Job drawing, mm, ordinate dimensions from the low corner. One solid piece. A direction names the side the tool comes from. Coordinates: 2 decimals unless noted, no trailing zeros. Loops run counter-clockwise (first coordinate to the right, second up) from the corner with the lowest first, then second, coordinate; pieces in that order, holes last. Notation, with made-up numbers: (24.5, 69) - (28.5, 69) arc R21 ccw to (28.5, 95) - close; hole circle Ø6 at (36.25, 73). An arc over 180 degrees is marked (long way). Use a Markdown table: item, result. Add a question column.
1. 3-axis set-ups, long thin cutter, end or side, ignore diameter. For the marked faces 5, 6, 7, 8 and 9: which of +Z, -Z, +X, -X, +Y, -Y reach the whole face in a straight line?
2. Band-saw the part on A-A, the plane x = 14.5. Give the cut face in (y, z).
3. Band-saw the part on C-C, the plane y = 13.5. Give the cut face in (x, z).
4. Pull direction Z, two halves, no side cores. Call the marked faces 1, 2, 3 and 4: pulls with the +Z half, pulls with the -Z half, needs draft (parallel to the pull), parting line crosses it, or undercut.
5. Band-saw the part on D-D, the plane z = 7.5. Give the cut face in (x, y), plus the area to 3 significant figures.
6. Band-saw the part on B-B, the plane y = 45. Give the cut face in (x, z), plus the area to 3 significant figures.
7. Wall check: probe 1 along Z at (x, y) = (26, 45); probe 2 along Z at (x, y) = (10, 29); probe 3 along X at (y, z) = (7.5, 12). Give the ranges that are in metal, low to high. Write a range as [from, to].
8. Drop flat-ended pins along their axis: pin 1 (3.5 mm diameter, centred on x = 6, y = 42.5, fed in from +Z); pin 2 (17.5 mm diameter, centred on y = 18, z = 27, fed in from -X); pin 3 (5.5 mm diameter, centred on x = 13.5, z = 18, fed in from -Y). Give the stop position or say it passes through.
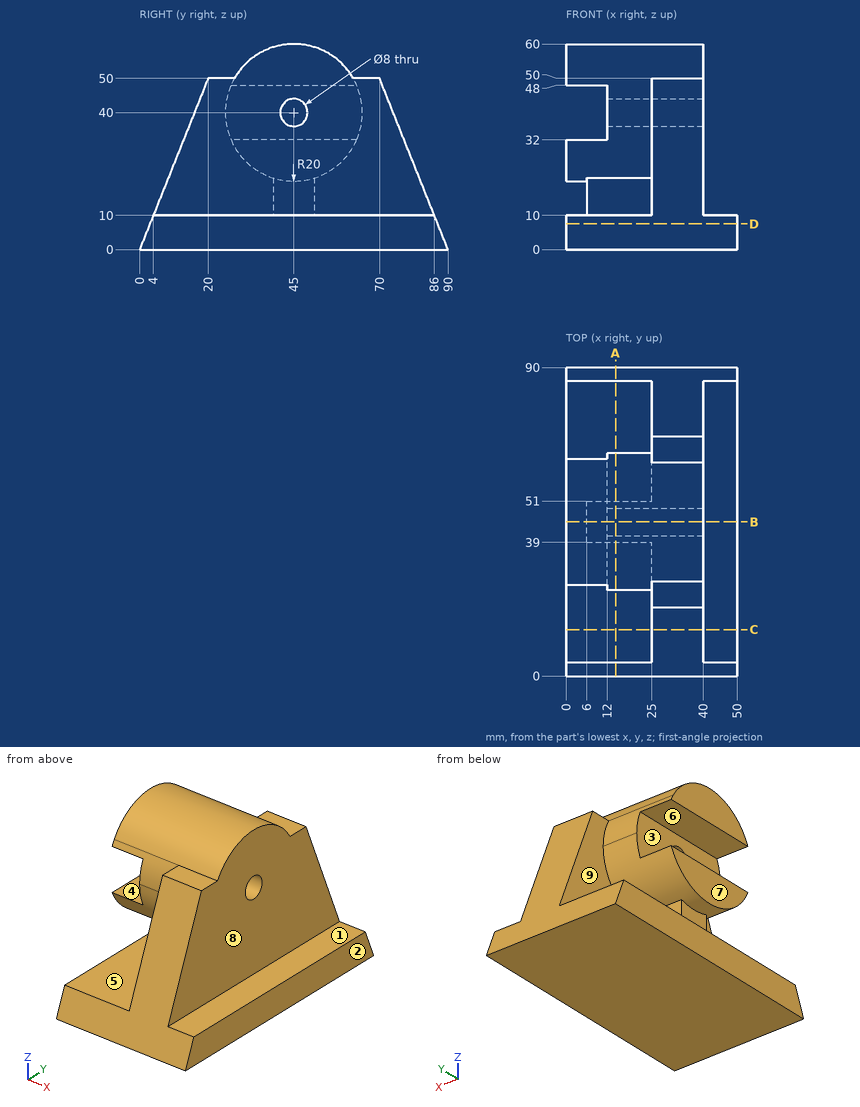
Geometry check:
| question | item | result |
|---|---|---|
| 1 | face 5 | -X |
| 1 | face 6 | -X, +Y, -Y |
| 1 | face 7 | +Z, -Z, -X, +Y, -Y |
| 1 | face 8 | +Z, +X, +Y, -Y |
| 1 | face 9 | -X, +Y |
| 2 | outline | (0, 0) - (90, 0) - (86, 10) - (51, 10) - (51, 20.92) arc R20 ccw (long way) to (39, 20.92) - (39, 10) - (4, 10) - close; hole circle Ø8 at (45, 40) |
| 3 | outline | (0, 0) - (50, 0) - (50, 10) - (40, 10) - (40, 33.75) - (25, 33.75) - (25, 10) - (0, 10) - close |
| 4 | face 1 | pulls with the +Z half |
| 4 | face 2 | needs draft |
| 4 | face 3 | undercut |
| 4 | face 4 | undercut |
| 5 | outline | (0, 3) - (50, 3) - (50, 87) - (0, 87) - close |
| 5 | area | 4,200 mm^2 |
| 6 | outline | (0, 0) - (50, 0) - (50, 10) - (40, 10) - (40, 36) - (12, 36) - (12, 32) - (0, 32) - (0, 20) - (6, 20) - (6, 10) - (0, 10) - close; (0, 48) - (12, 48) - (12, 44) - (40, 44) - (40, 60) - (0, 60) - close |
| 6 | area | 2,020 mm^2 |
| 7 | probe 1 | z = [0, 36], [44, 60] |
| 7 | probe 2 | z = [0, 10], [28, 32], [48, 52] |
| 7 | probe 3 | x = [25, 40] |
| 8 | pin 1 | stops at z = 59.99 |
| 8 | pin 2 | stops at x = 25 |
| 8 | pin 3 | stops at y = 39 |
